Autodesk Inventor part; units mm, degrees
ref_plane "YZ Plane" through (0, 0, 0) normal (1, 0, 0) x (0, 1, 0)
ref_plane "XZ Plane" through (0, 0, 0) normal (0, 1, 0) x (-1, 0, 0)
ref_plane "XY Plane" through (0, 0, 0) normal (0, 0, 1) x (1, 0, 0)
sketch "Sketch1" plane through (0, 0, 0) normal (0, 1, 0) x (-1, 0, 0)
  circle A0 centre (0, 0) radius 22.5044
  dimension "d0" = 45.0088
extrude "Extrusion1" add sketch "Sketch1" along normal blind 50.8
sketch "Sketch4" plane through (0, 50.8, 0) normal (0, 1, 0) x (1, 0, 0)
  circle A0 centre (15.24, 0) radius 3.175
  circle A1 centre (0, 15.24) radius 3.175
  circle A2 centre (-15.24, 0) radius 3.175
  circle A3 centre (0, -15.24) radius 3.175
  point P0 (0, 0)
  dimension "d6" = 6.35
  dimension "d7" = 0
  dimension "d8" = 15.24
  dimension "d11" = 360
extrude "Extrusion3" cut sketch "Sketch4" against normal blind 25.4
properties part number "FrontPlatePostNoKey"
Input: part model. Units: mm. Frame: model coordinates. A direction names the side the tool comes from. Give positions to 0.01 mm unless a question says otherwise; leave off trailing zeros. Order: outer loops, then holes, each group sorted by start corner. A loop starts at its lowest first (then second) coordinate and runs counter-clockwise, first axis right, second up. Notation, with made-up numbers: M 3.5,76 L 12.5,76 A22 ccw 12.5,86 Z; hole C 3.25,23.25 d2. An arc over 180 degrees is marked long. One line per question, with ' | ' between items. Start each with the question number.
1. Section query D-D (y = 17). Return the cut outline in (x, z), and give its area (3 significant figures).
2. Section query C-C (x = 15.24). Return the cut outline in (y, z) (3 decimals), and give its area (3 significant figures).
3. Pull-direction query (Z, two-part tool) for faces 3 (the face through (2.93, 25.044, -22.313)), 4 (the face through (12.07, 38.28, -0.14)), 5 (the face through (0, 50.8, 0)); classes: released by +Z, released by -Z, zero draft, split by the parting line, or undercut.
4. Section query B-B (z = 0). Return the cut outline in (x, y) (3 decimals).
5. Access query for faces 1 (the face through (-0.69, 38.28, -12.14)), 2 (the face through (0, 0, 0)). Directions: +Z, -Z, +X, -X, +Y, -Y. A direction counts if a zero-diameter tool reaches every point of the face in a straight line with its end or side. Return the directions, or none.
6. First-contact query: pin 1 Ø4 at (x, z) = (0, -15.24) entering from +Y; pin 2 Ø10 at (x, y) = (-17, 45.5) entering from +Z; pin 3 Ø6 at (y, z) = (19, -16.5) entering from -X. Flat tips, straight axial feed; report the tip coordinate or a pass-through.
7. Section query A-A (y = 40.5). Return the cut outline in (x, z) (3 decimals), and give its area (3 significant figures).
8. Material intervals for probe 1 along Z at (x, y) = (0, 35.75) (3 decimals); probe 2 along Z at (x, y) = (13, 41); probe 3 along X at (y, z) = (35.5, -15.24) (3 decimals), sorted ascending. Write a range as [from, to].
Here are the results:
1) outline: C 0,0 d45.01 | area: 1,590 mm²
2) outline: M 0,-16.559 L 50.8,-16.559 L 50.8,-3.175 L 25.4,-3.175 L 25.4,3.175 L 50.8,3.175 L 50.8,16.559 L 0,16.559 Z | area: 1,520 mm²
3) face 3: split by the parting line | face 4: undercut | face 5: zero draft
4) outline: M -22.504,0 L 22.504,0 L 22.504,50.8 L 18.415,50.8 L 18.415,25.4 L 12.065,25.4 L 12.065,50.8 L -12.065,50.8 L -12.065,25.4 L -18.415,25.4 L -18.415,50.8 L -22.504,50.8 Z
5) face 1: +Y | face 2: +Z, -Z, +X, -X, -Y
6) pin 1: y = 25.4 | pin 2: z = 19.04 | pin 3: x = -18.01
7) outline: C 0,0 d45.009; hole C -15.24,0 d6.35; hole C 0,-15.24 d6.35; hole C 0,15.24 d6.35; hole C 15.24,0 d6.35 | area: 1,460 mm²
8) probe 1: [-22.504, -18.415], [-12.065, 12.065], [18.415, 22.504] | probe 2: [-18.37, -2.25], [2.25, 18.37] | probe 3: [-16.559, -3.175], [3.175, 16.559]
